Work out the finished part from the listing and answer in its coordinate system (mm). A direction names the side the tool comes from. Round coordinates to 2 decimals unless told otherwise and drop trailing zeros. Write each loop counter-clockwise with the first axis right and the second up, starting at its lowest first coordinate (ties: lowest second). Pieces come first, ordered by that corner, then holes. Notation, with made-up numbers: M 8,-11 L 40,-11 A18 ccw 40,12 Z; hole C 28.5,58 d8. An arc over 180 degrees is marked long. Answer in a Markdown table with one row per item.
```python
from build123d import *

# Parameters (mm, degrees)
F0_R      = 25
F0_R_2    = 21
F1_DEPTH  = 10
F2_R      = 25
F3_DEPTH  = 10
F4_R      = 25
F4_R_2    = 21
F5_DEPTH  = 320
F6_R      = 25
F7_DEPTH  = 10
F8_R      = 5
F9_DEPTH  = 10
F10_R     = 5
F11_DEPTH = 10


with BuildPart() as f1:
    # F0 (on Top) → F1 (new body)
    with BuildSketch(Plane.XY):
        Circle(F0_R)
        Circle(F0_R_2, mode=Mode.SUBTRACT)
    extrude(amount=F1_DEPTH)

    # F2 (on face) → F3 (join)
    with BuildSketch(Plane.XY.offset(10)):
        Circle(F2_R)
    extrude(amount=F3_DEPTH)

    # F4 (on face) → F5 (join)
    with BuildSketch(Plane.XY.offset(20)):
        Circle(F4_R)
        Circle(F4_R_2, mode=Mode.SUBTRACT)
    extrude(amount=F5_DEPTH)

    # F6 (on face) → F7 (join)
    with BuildSketch(Plane.XY.offset(340)):
        Circle(F6_R)
    extrude(amount=F7_DEPTH)

    # F8 (on face) → F9 (cut)
    with BuildSketch(Plane(origin=(0, 0, 10), x_dir=(1, 0, 0), z_dir=(0, 0, -1))):
        Circle(F8_R)
    extrude(amount=-F9_DEPTH, mode=Mode.SUBTRACT)

    # F10 (on face) → F11 (cut)
    with BuildSketch(Plane.XY.offset(350)):
        Circle(F10_R)
    extrude(amount=-F11_DEPTH, mode=Mode.SUBTRACT)


solid = f1.part
```
1. Determine the mould class of faces 3 (the flat face through (4, -4, 10)), 4 (the flat face through (4, -4, 340)), 5 (the cylindrical face through (20.03, 6.31, 4.93)) for opening direction Z: released by +Z, released by -Z, zero draft, split by the parting line, or undercut.
Calculated:
| item | result |
|---|---|
| face 3 | released by -Z |
| face 4 | undercut |
| face 5 | zero draft |
2. The part is cut by section D-D (z = 136.5). Determine the outline of the cut face in (x, y), plus the area to 3 significant figures.
Calculated:
| item | result |
|---|---|
| outline | C 0,0 d50; hole C 0,0 d42 |
| area | 578 mm² |
3. The part is cut by section A-A (x = 0). Determine the outline of the cut face in (y, z).
Calculated:
| item | result |
|---|---|
| outline | M -25,0 L -21,0 L -21,10 L -5,10 L -5,20 L -21,20 L -21,340 L -5,340 L -5,350 L -25,350 Z; M 5,10 L 21,10 L 21,0 L 25,0 L 25,350 L 5,350 L 5,340 L 21,340 L 21,20 L 5,20 Z |
4. Given pin 1 (1.5 mm diameter, centred on x = -16, z = 168, fed in from +Y); pin 2 (1.5 mm diameter, centred on x = 2, z = 282.5, fed in from +Y); pin 3 (25 mm diameter, centred on x = 0, y = 0, fed in from +Z); pin 4 (6 mm diameter, centred on x = 0, y = 0, fed in from -Z), each flat-ended and moving along its own axis, determine where each tip first touches the part or whether it passes through.
Calculated:
| item | result |
|---|---|
| pin 1 | stops at y = 19.81 |
| pin 2 | stops at y = 24.97 |
| pin 3 | stops at z = 350 |
| pin 4 | passes through |
5. Consider line 1 along Z through (x, y) = (11, 16); line 2 along Y through (x, z) = (0, 139.5); line 3 along Y through (x, z) = (-9.5, 281). Determine where each line is inside the solid, lowest interval first. Write a range as from..to.
Calculated:
| item | result |
|---|---|
| line 1 | z = 10..20, 340..350 |
| line 2 | y = -25..-21, 21..25 |
| line 3 | y = -23.12..-18.73, 18.73..23.12 |
6. A tool of negligible diameter and unlimited length cuts with its end or side. For faces 1 (the flat face through (-5.7, 20.5, 0)), 2 (the cylindrical face through (20.03, 6.31, 177.76)), from which of +Z, -Z, +X, -X, +Y, -Y can it reach the whole face along a straight path? Write none if from no direction.
Calculated:
| item | result |
|---|---|
| face 1 | -Z, +X, -X, +Y, -Y |
| face 2 | none |
7. The part is cut by section C-C (y = -16.5). Determine the outline of the cut face in (x, z), plus the area to 3 significant figures.
Calculated:
| item | result |
|---|---|
| outline | M -18.78,0 L -12.99,0 L -12.99,10 L 12.99,10 L 12.99,0 L 18.78,0 L 18.78,350 L -18.78,350 Z; hole M -12.99,20 L 12.99,20 L 12.99,340 L -12.99,340 Z |
| area | 4,570 mm² |
